Can you work these out from the model? Positions are in its coordinate system, mm. A direction names the side the tool comes from. Give positions to 0.01 mm unless a question says otherwise; leave off trailing zeros. Write each loop counter-clockwise with the first axis right and the second up, starting at its lowest first coordinate (ties: lowest second). Pieces come first, ordered by that corner, then holes. Notation, with made-up numbers: (49.5, 46.5) -> (91.5, 46.5) arc R13 ccw to (91.5, 68.5) -> close; hole circle Ø6 at (54.5, 41). An arc over 180 degrees is marked (long way). One line per item, written item: value.
from build123d import *

# Parameters (mm, degrees)
BOSS_EXTRUDE1_DEPTH = 10
FILLET1_R           = 2
SKETCH4_R           = 2.6
CUT_EXTRUDE2_DEPTH  = 50.150169347


with BuildPart() as part:
    # Sketch1 → Boss-Extrude1 (new body)
    with BuildSketch(Plane.XY):
        with BuildLine():
            Line((10, 0), (25, 0))
            Line((25, 0), (25, 14))
            Line((25, 14), (33, 14))
            Line((33, 14), (33, 11.313708499))
            ThreePointArc((33, 11.313708499), (37.561789374, 11.986842482), (42.040624961, 10.89))
            Line((42.040624961, 10.89), (46.040624961, 10.89))
            Line((46.040624961, 10.89), (46.040624961, 8.636671813))
            Line((46.040624961, 8.636671813), (42.040624961, 8.636671813))
            ThreePointArc((42.040624961, 8.636671813), (27, 0), (42.040624961, -8.636671813))
            Line((42.040624961, -8.636671813), (46.040624961, -8.636671813))
            Line((46.040624961, -8.636671813), (46.040624961, -10.89))
            Line((46.040624961, -10.89), (42.040624961, -10.89))
            ThreePointArc((42.040624961, -10.89), (37.561789374, -11.986842482), (33, -11.313708499))
            Line((33, -11.313708499), (33, -14))
            Line((33, -14), (25, -14))
            Line((25, -14), (-25, -14))
            Line((-25, -14), (-25, 0))
            Line((-25, 0), (-10, 0))
            ThreePointArc((-10, 0), (0, -10), (10, 0))
        make_face()
    extrude(amount=BOSS_EXTRUDE1_DEPTH)

    # Fillet1
    fillet1_edges = [part.edges().sort_by_distance(p)[0] for p in [
        (-25, -7, 10),
        (-25, -7, 0),
        (33, 11.313708499, 5),
        (42.040624961, 10.89, 5),
        (46.040624961, 8.636671813, 5),
        (46.040624961, -8.636671813, 5),
        (42.040624961, -10.89, 5),
        (33, -11.313708499, 5),
    ]]
    fillet(fillet1_edges, radius=FILLET1_R)

    # Sketch4 → Cut-Extrude2 (cut, through all)
    with BuildSketch(Plane(origin=(0, 0, 0), x_dir=(1, 0, 0), z_dir=(0, 1, 0))):
        with Locations(Location((-17, -5, 0), (0, 0, 180))):
            Circle(SKETCH4_R)
        with Locations(Location((17, -5, 0), (0, 0, 180))):
            Circle(SKETCH4_R)
    extrude(amount=-CUT_EXTRUDE2_DEPTH, mode=Mode.SUBTRACT)


solid = part.part
1) For faces 1 (the face through (-19, 0, 3)), 2 (the face through (44, 10.89, 5)), 3 (the face through (44, -10.89, 5)), 4 (the face through (43, 8.637, 5)), which set-ups out of +Z, -Z, +X, -X, +Y, -Y let a thin tool reach every point of the face, with its end or its side?
Answer list:
face 1: +Z, -Z, -X, +Y
face 2: +Z, -Z, +X, +Y
face 3: +Z, -Z, +X, -Y
face 4: +Z, -Z, +X
2) I need wall thicknesses on L1, parallel to Z at x = -17, y = -7.25; L2, parallel to Y at x = 37, z = 2.5; L3, parallel to Z at x = 19, y = -10.5. Which ranges of each line are inside material? Lowest first, please.
Answer list:
L1: z = 0 to 2.4, 7.6 to 10
L2: y = -12 to -10, 10 to 12
L3: z = 0 to 3.34, 6.66 to 10
3) If we section it at D-D (x = -8): Write out the boundary of the cut face in (y, z), and give its area (3 significant figures).
Answer list:
outline: (-14, 0) -> (-6, 0) -> (-6, 10) -> (-14, 10) -> close
area: 80.0 mm^2
4) If we section it at B-B (x = -17): Write out the boundary of the cut face in (y, z).
Answer list:
outline: (-14, 0) -> (0, 0) -> (0, 2.4) -> (-14, 2.4) -> close; (-14, 7.6) -> (0, 7.6) -> (0, 10) -> (-14, 10) -> close
5) If we section it at A-A (y = -6): Write out the boundary of the cut face in (x, z).
Answer list:
outline: (-25, 2) arc R2 ccw to (-23, 0) -> (-8, 0) -> (-8, 10) -> (-23, 10) arc R2 ccw to (-25, 8) -> close; (8, 0) -> (29, 0) -> (29, 10) -> (8, 10) -> close; hole circle Ø5.2 at (-17, 5); hole circle Ø5.2 at (17, 5)
6) Will these pins go through, and if not, where does the flat tip stop? pin 1 (5 mm diameter, centred on y = -11, z = 7.5, fed in from +X); pin 2 (1.6 mm diameter, centred on x = 43, z = 6, fed in from +Y); pin 3 (3 mm diameter, centred on x = 44.5, z = 7.5, fed in from -Y); pin 4 (3 mm diameter, centred on x = -17, z = 5, fed in from -Y).
Answer list:
pin 1: stops at x = 46.04
pin 2: stops at y = 10.91
pin 3: stops at y = -10.89
pin 4: passes through
7) If we section it at C-C (z = 3.25): State how many separate pieces and enclosed holes the cut face has, and give its area (3 significant figures).
Answer list:
separate pieces: 3
enclosed holes: 0
area: 636 mm^2
8) We'd pull the mould along X, two halves only. Please class faces 5 (the face through (45.47, 9.24, 5.07)), 6 (the face through (33.71, -12.33, 5.07)), 7 (the face through (19, 0, 3)), 8 (the face through (-24.43, -6.9, 0.6)): released by +X, released by -X, zero draft, split by the parting line, or undercut.
Answer list:
face 5: released by +X
face 6: undercut
face 7: zero draft
face 8: released by -X
